Can you work these out from the model? Positions are in its coordinate system, mm. A direction names the side the tool comes from. Coordinates: 2 decimals unless noted, no trailing zeros. Write each loop counter-clockwise with the first axis right and the second up, starting at its lowest first coordinate (ties: lowest second). Pieces come first, ordered by that corner, then holes. Notation, with made-up numbers: (82, 73) -> (106, 73) arc R23 cw to (106, 108) -> close; hole circle Ø5 at (-35, 22). An arc over 180 degrees is marked (long way). Use one line per item in the form item = value.
```python
from build123d import *

# Parameters (mm, degrees)
F0_W     = 155
F0_H     = 47
F1_DEPTH = 77
F2_W     = 103
F2_H     = 38
F2_W_2   = 37
F3_DEPTH = 75
F5_DEPTH = 3
F6_W     = 5
F6_H     = 3
F7_DEPTH = 75


with BuildPart() as f1:
    # F0 (on Top) → F1 (new body)
    with BuildSketch(Plane.XY):
        Rectangle(F0_W, F0_H)
    extrude(amount=F1_DEPTH)

    # F2 (on face) → F3 (cut)
    with BuildSketch(Plane.XY.offset(77)):
        with Locations((-21, 0.5)):
            Rectangle(F2_W, F2_H)
        with Locations((54, 0.5)):
            Rectangle(F2_W_2, F2_H)
    extrude(amount=-F3_DEPTH, mode=Mode.SUBTRACT)

    # F4 (on face) → F5 (cut)
    with BuildSketch(Plane.XZ.offset(23.5)):
        Polygon((-77.5, 38.5), (0, 77), (-11.2384570943, 77), (-77.5, 44.0829754598), align=None)
        Polygon((0, 0), (-77.5, 38.5), (-77.5, 32.9170245402), (-11.2384570943, 0), align=None)
        Polygon((77.5, 32.9170245402), (77.5, 38.5), (0, 0), (11.2384570943, 0), align=None)
        Polygon((11.2384570943, 77), (0, 77), (77.5, 38.5), (77.5, 44.0829754598), align=None)
    extrude(amount=-F5_DEPTH, mode=Mode.SUBTRACT)

    # F6 (on face) → F7 (cut)
    with BuildSketch(Plane.XY.offset(77)):
        with Locations((50, -20)):
            Rectangle(F6_W, F6_H)
        with Locations((25, -20)):
            Rectangle(F6_W, F6_H)
        with Locations((-25, -20)):
            Rectangle(F6_W, F6_H)
        with Locations((-50, -20)):
            Rectangle(F6_W, F6_H)
    extrude(amount=-F7_DEPTH, mode=Mode.SUBTRACT)


solid = f1.part
```
Q1. If I drill on line 1 (X direction, y = -6.5, z = 5); line 2 (Y direction, x = -19.5, z = 69); line 3 (Y direction, x = -59, z = 70), over which ranges is the centre line in solid material (lowest first)? Write a range as from..to.
Return value:
line_1 = -77.5..-72.5, 30.5..35.5, 72.5..77.5
line_2 = -20.5..-18.5, 19.5..23.5
line_3 = -23.5..-18.5, 19.5..23.5
Q2. Suppose I cut it at C-C (x = -13.5). Write out the boundary of the cut face in (y, z), then the cut area to 4 significant figures.
Return value:
outline = (-23.5, 0) -> (23.5, 0) -> (23.5, 77) -> (19.5, 77) -> (19.5, 2) -> (-18.5, 2) -> (-18.5, 77) -> (-23.5, 77) -> (-23.5, 75.88) -> (-20.5, 75.88) -> (-20.5, 70.29) -> (-23.5, 70.29) -> (-23.5, 6.71) -> (-20.5, 6.71) -> (-20.5, 1.12) -> (-23.5, 1.12) -> close
area = 735.5 mm2
Q3. Suppose I cut it at B-B (x = 25.5). Write out the boundary of the cut face in (y, z), then the cut area to 3 significant figures.
Return value:
outline = (-23.5, 0) -> (23.5, 0) -> (23.5, 77) -> (19.5, 77) -> (19.5, 2) -> (-21.5, 2) -> (-21.5, 7.08) -> (-23.5, 7.08) -> close; (-23.5, 12.67) -> (-21.5, 12.67) -> (-21.5, 64.33) -> (-23.5, 64.33) -> close; (-23.5, 69.92) -> (-21.5, 69.92) -> (-21.5, 77) -> (-23.5, 77) -> close
area = 522 mm2
Q4. For faces 1 (the flat face through (50, -21.5, 39)), 2 (the flat face through (-1, 0, 0)), 3 (the flat face through (44.833, -22.021, 60.311)), which set-ups out of +Z, -Z, +X, -X, +Y, -Y let a thin tool reach every point of the face, with its end or its side?
Return value:
face_1 = +Z
face_2 = -Z, +X, -X, +Y, -Y
face_3 = -Y
Q5. Will this pin go through, and if not, where does the flat tip stop? pin 1 (1.5 mm diameter, centred on x = -4, y = 18, fed in from +Z).
Return value:
pin_1 = 2
Q6. Suppose I cut it at A-A (y = 2.5). Write out the boundary of the cut face in (x, z), then the cut area to 4 significant figures.
Return value:
outline = (-77.5, 0) -> (77.5, 0) -> (77.5, 77) -> (72.5, 77) -> (72.5, 2) -> (35.5, 2) -> (35.5, 77) -> (30.5, 77) -> (30.5, 2) -> (-72.5, 2) -> (-72.5, 77) -> (-77.5, 77) -> close
area = 1,435 mm2
Q7. Thinking about a two-plate mould opening in Z: for faces 4 (the flat face through (-50, -21.5, 67)), 5 (the flat face through (5, -19, 77)), 6 (the flat face through (38.21, -22.02, 58.02)), 7 (the flat face through (-38, -20.5, 16)), which applies, released by +Z, released by -Z, zero draft, split by the parting line, or undercut?
Return value:
face_4 = zero draft
face_5 = released by +Z
face_6 = undercut
face_7 = undercut
Q8. Suppose I cut it at D-D (z = 60.5). Give the number of separate pieces and of enclosed holes in the cut face, then the cut area to 3 significant figures.
Return value:
separate_pieces = 1
enclosed_holes = 2
area = 1,840 mm2
